Input: dimensioned drawing with shaded views. Units: mm. Origin: part minimum x, y, z. Coordinates: 2 decimals unless noted, no trailing zeros. Write each loop counter-clockwise with the first axis right and the second up, starting at its lowest first coordinate (ties: lowest second). Pieces come first, ordered by that corner, then holes. Notation, with made-up numbers: (-31.75, 18.5) -> (7.25, 18.5) arc R37 ccw to (7.25, 57.5) -> close; hole circle Ø1 at (42.25, 78.5). An arc over 180 degrees is marked (long way). One line per item, written item: value. Start each with the question number.
1. Section query D-D, the plane z = 33.5. Output: boundary loops of the cut face in (x, y).
2. Section query B-B, the plane y = 13.5. Output: boundary loops of the cut face in (x, z).
3. Line query: line 1 (Y direction, x = 55, z = 36.25); line 2 (Z direction, x = 46.5, y = 25); line 3 (X direction, y = 17, z = 23). Output: solid intervals per line, ascending.
4. Section query A-A, the plane x = 31. Output: boundary loops of the cut face in (y, z).
5. First-contact query: P1, Ø1.8, axis at x = 5.5, y = 8, coming from the +Z side; P2, Ø5, axis at x = 7, y = 32, coming from the -Z side. Flat tips, straight axial feed; report the tip coordinate or a pass-through.
6. Section query C-C, the plane z = 15.5. Output: boundary loops of the cut face in (x, y), and give its area (3 significant figures).
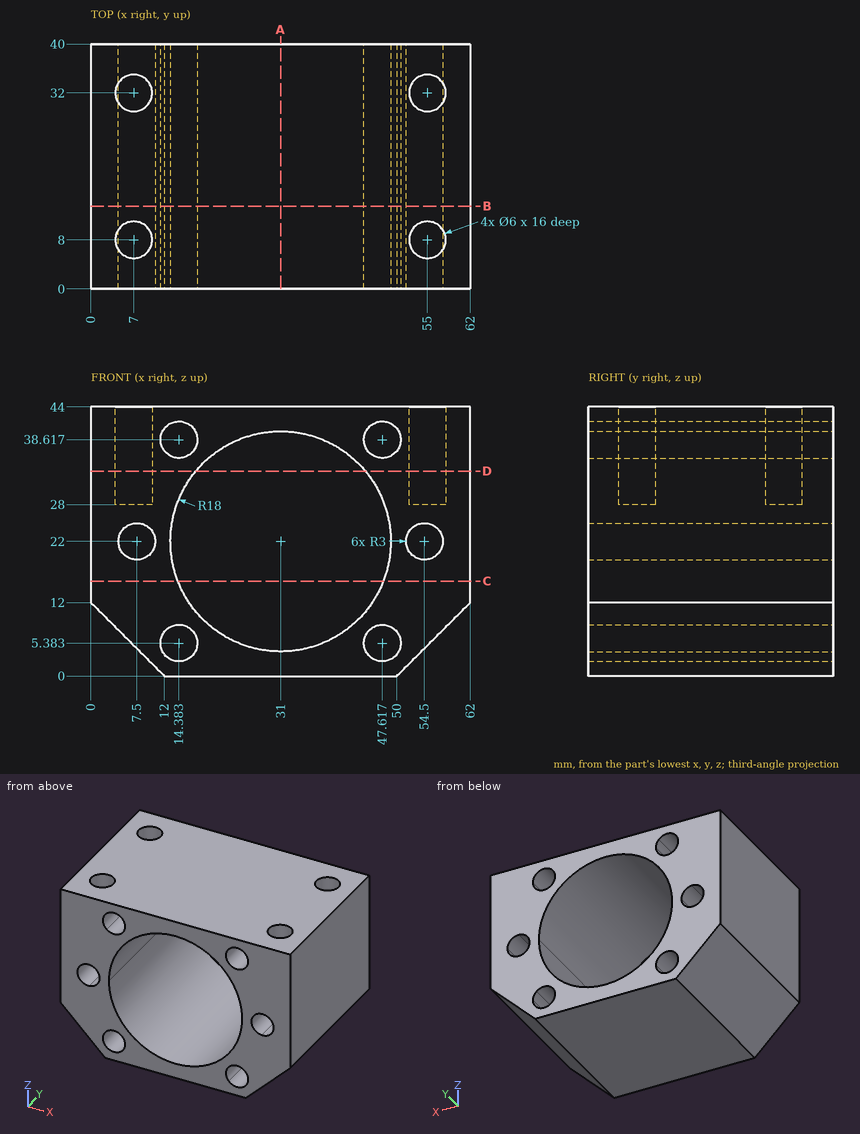
Computed values:
1. outline: (0, 0) -> (17.15, 0) -> (17.15, 40) -> (0, 40) -> close; (44.85, 0) -> (62, 0) -> (62, 40) -> (44.85, 40) -> close; hole circle Ø6 at (7, 8); hole circle Ø6 at (7, 32); hole circle Ø6 at (55, 8); hole circle Ø6 at (55, 32)
2. outline: (0, 12) -> (12, 0) -> (50, 0) -> (62, 12) -> (62, 44) -> (0, 44) -> close; hole circle Ø6 at (7.5, 22); hole (13, 22) arc R18 ccw (long way) to (18.27, 34.73) arc R18 ccw to start; hole (16.5, 36.5) arc R3 ccw to (17.38, 38.62) arc R3 ccw to (16.64, 40.6) arc R3 ccw (long way) to start; hole (16.64, 3.4) arc R3 ccw to (17.38, 5.38) arc R3 ccw (long way) to start; hole (49.6, 7.64) arc R3 ccw (long way) to (50.62, 5.38) arc R3 ccw to start; hole (49.6, 36.36) arc R3 ccw to (50.62, 38.62) arc R3 ccw (long way) to start; hole circle Ø6 at (54.5, 22)
3. line 1: y = 0 to 5, 11 to 29, 35 to 40
3. line 2: z = 0 to 2.6, 8.17 to 12.85, 31.15 to 35.83, 41.4 to 44
3. line 3: x = 0 to 4.67, 10.33 to 13.03, 48.97 to 51.67, 57.33 to 62
4. outline: (0, 0) -> (40, 0) -> (40, 4) -> (0, 4) -> close; (0, 40) -> (40, 40) -> (40, 44) -> (0, 44) -> close
5. P1: stops at z = 28
5. P2: stops at z = 2.5
6. outline: (0, 0) -> (14.21, 0) -> (14.21, 40) -> (0, 40) -> close; (47.79, 0) -> (62, 0) -> (62, 40) -> (47.79, 40) -> close
6. area: 1,140 mm²
